Model file for the job. Use its own axes, mm. Round coordinates to 2 decimals unless told otherwise and drop trailing zeros. Order: outer loops, then holes, each group sorted by start corner. A loop starts at its lowest first (then second) coordinate and runs counter-clockwise, first axis right, second up. Notation, with made-up numbers: M 41.5,32 L 77.5,32 A30 ccw 77.5,60 Z; hole C 6.25,50.5 d4. An arc over 180 degrees is marked long. Return JSON: item names as keys, results as strings. Group by question number.
Item 1: Slice it at A-A on x = 0. Write the cut outline in (y, z), then the cut area to 3 significant figures.
Item 2: Slice it at C-C on z = 0. Write the cut outline in (x, y).
Item 3: Slice it at B-B on y = 0. Write the cut outline in (x, z), then the cut area to 3 significant figures.
Item 4: Probe line 1 along Y through (x, z) = (-29, 0); line 2 along Y through (x, z) = (0, 7.5). List the from-to ranges inside material, lowest first.
Item 5: Pin check, flat tips, straight feed: pin 1 Ø10 at (x, y) = (5, 4.5) entering from -Z; pin 2 Ø9 at (y, z) = (0, 0) entering from -X. Stop position of each tip, or through.
Item 6: Pull direction Y, two halves, no side cores. Call faces 1 (the face through (9, 0, 15)), 2 (the face through (-1, -15, 0)), 3 (the face through (-0.976, 7.436, -0.21)): pulls with the +Y half, pulls with the -Y half, needs draft (parallel to the pull), parting line crosses it, or undercut.
Item 7: Slice it at D-D on z = 7. Write the cut outline in (x, y), then the cut area to 3 significant figures.
from build123d import *

# Parameters (mm, degrees)
CROQUIS1_W              = 86
CROQUIS1_H              = 30
CROQUIS1_R              = 7.5
SALIENTE_EXTRUIR1_DEPTH = 15
CROQUIS2_R              = 5
CORTAR_EXTRUIR1_DEPTH   = 87


with BuildPart() as part:
    # Croquis1 → Saliente-Extruir1 (new body, symmetric)
    with BuildSketch(Plane.XY):
        Rectangle(CROQUIS1_W, CROQUIS1_H)
        Circle(CROQUIS1_R, mode=Mode.SUBTRACT)
    extrude(amount=SALIENTE_EXTRUIR1_DEPTH, both=True)

    # Croquis2 → Cortar-Extruir1 (cut, through all)
    with BuildSketch(Plane(origin=(43, 0, 0), x_dir=(0, 0, -1), z_dir=(1, 0, 0))):
        Circle(CROQUIS2_R)
    extrude(amount=-CORTAR_EXTRUIR1_DEPTH, mode=Mode.SUBTRACT)


solid = part.part
Output values:
{
 "1": {"outline": "M -15,-15 L -7.5,-15 L -7.5,15 L -15,15 Z; M 7.5,-15 L 15,-15 L 15,15 L 7.5,15 Z", "area": "450 mm²"},
 "2": {"outline": "M -43,-15 L 43,-15 L 43,-5 L 5.59,-5 A7.5 cw -5.59,-5 L -43,-5 Z; M -43,5 L -5.59,5 A7.5 cw 5.59,5 L 43,5 L 43,15 L -43,15 Z"},
 "3": {"outline": "M -43,-15 L -7.5,-15 L -7.5,-5 L -43,-5 Z; M -43,5 L -7.5,5 L -7.5,15 L -43,15 Z; M 7.5,-15 L 43,-15 L 43,-5 L 7.5,-5 Z; M 7.5,5 L 43,5 L 43,15 L 7.5,15 Z", "area": "1,420 mm²"},
 "4": {"line 1": "-15 to -5, 5 to 15", "line 2": "-15 to -7.5, 7.5 to 15"},
 "5": {"pin 1": "z = -15", "pin 2": "through"},
 "6": {"face 1": "needs draft", "face 2": "pulls with the -Y half", "face 3": "undercut"},
 "7": {"outline": "M -43,-15 L 43,-15 L 43,15 L -43,15 Z; hole C 0,0 d15", "area": "2,400 mm²"}
}
